from build123d import *

# Parameters (mm, degrees)
SKETCH_1_W                  = 320
SKETCH_1_H                  = 210
SKETCH_1_W_2                = 50
EXTRUDE_1_DEPTH             = 5
HOLE_WIZARD_M61_AT_2_COUNT  = 2
HOLE_WIZARD_M61_AT_2_PITCH  = 258
HOLE_WIZARD_M61_AT_3_COUNT  = 2
HOLE_WIZARD_M61_AT_3_PITCH  = 75
HOLE_WIZARD_M61_AT_4_COUNT  = 2
HOLE_WIZARD_M61_AT_4_PITCH  = 268.680107191
HOLE_WIZARD_M61_AT_5_COUNT  = 2
HOLE_WIZARD_M61_AT_5_PITCH  = 150
HOLE_WIZARD_M61_AT_6_COUNT  = 2
HOLE_WIZARD_M61_AT_6_PITCH  = 298.435922771
HOLE_WIZARD_M61_AT_7_COUNT  = 2
HOLE_WIZARD_M61_AT_7_PITCH  = 225
HOLE_WIZARD_M61_AT_8_COUNT  = 2
HOLE_WIZARD_M61_AT_8_PITCH  = 342.328789324
HOLE_WIZARD_M61_AT_9_COUNT  = 2
HOLE_WIZARD_M61_AT_9_PITCH  = 300
HOLE_WIZARD_M61_AT_10_COUNT = 2
HOLE_WIZARD_M61_AT_10_PITCH = 395.681690251
HOLE_WIZARD_M61_AT_11_COUNT = 2
HOLE_WIZARD_M61_AT_11_PITCH = 375
HOLE_WIZARD_M61_AT_12_COUNT = 2
HOLE_WIZARD_M61_AT_12_PITCH = 455.180184103
HOLE_WIZARD_M61_AT_13_COUNT = 2
HOLE_WIZARD_M61_AT_13_PITCH = 450
HOLE_WIZARD_M61_AT_14_COUNT = 2
HOLE_WIZARD_M61_AT_14_PITCH = 518.713793917
HOLE_WIZARD_M61_AT_15_COUNT = 2
HOLE_WIZARD_M61_AT_15_PITCH = 525
HOLE_WIZARD_M61_AT_16_COUNT = 2
HOLE_WIZARD_M61_AT_16_PITCH = 584.96922996
HOLE_WIZARD_M61_AT_17_COUNT = 2
HOLE_WIZARD_M61_AT_17_PITCH = 600
HOLE_WIZARD_M61_AT_18_COUNT = 2
HOLE_WIZARD_M61_AT_18_PITCH = 653.118672218
HOLE_WIZARD_M61_AT_19_COUNT = 2
HOLE_WIZARD_M61_AT_19_PITCH = 675
HOLE_WIZARD_M61_AT_20_COUNT = 2
HOLE_WIZARD_M61_AT_20_PITCH = 722.626459521
HOLE_WIZARD_M62_AT_2_COUNT  = 2
HOLE_WIZARD_M62_AT_2_PITCH  = 598
HOLE_WIZARD_M62_AT_3_COUNT  = 2
HOLE_WIZARD_M62_AT_3_PITCH  = 750
HOLE_WIZARD_M62_AT_4_COUNT  = 2
HOLE_WIZARD_M62_AT_4_PITCH  = 75
HOLE_WIZARD_M62_AT_5_COUNT  = 2
HOLE_WIZARD_M62_AT_5_PITCH  = 602.684826423
HOLE_WIZARD_M62_AT_6_COUNT  = 2
HOLE_WIZARD_M62_AT_6_PITCH  = 753.740671584
HOLE_WIZARD_M62_AT_7_COUNT  = 2
HOLE_WIZARD_M62_AT_7_PITCH  = 150
HOLE_WIZARD_M62_AT_8_COUNT  = 2
HOLE_WIZARD_M62_AT_8_PITCH  = 616.525749665
HOLE_WIZARD_M62_AT_9_COUNT  = 2
HOLE_WIZARD_M62_AT_9_PITCH  = 764.852927039


with BuildPart() as part:
    # Эскиз1 → Бобышка-Вытянуть1 (new body)
    with BuildSketch(Plane.XY):
        Polygon((0, 0), (750, 0), (750, 298), (0, 298), (-40, 298), (-40, 0), align=None)
        with Locations((394, 149)):
            Rectangle(SKETCH_1_W, SKETCH_1_H, mode=Mode.SUBTRACT)
        with Locations((189, 149)):
            Rectangle(SKETCH_1_W_2, SKETCH_1_H, mode=Mode.SUBTRACT)
    extrude(amount=EXTRUDE_1_DEPTH)

    # Эскиз2 → Зенковка для винта с потайной головкой и внутренним шестигранником M61 (revolve, cut)
    with BuildSketch(Plane(origin=(37.5, 278, 5), x_dir=(0, -1, 0), z_dir=(1, 0, 0))):
        Polygon((0, 0), (0, 5), (3.3, 5), (3.3, 3.555), (6.855, 0), align=None)
    hole_wizard_m61 = revolve(axis=Axis((37.5, 278, 11.35), (0, 0, -1)), mode=Mode.SUBTRACT)

    # Зенковка для винта с потайной головкой и внутренним шестигранником M61 at 2: Зенковка для винта с потайной головкой и внутренним шестигранником M61 ×2
    with Locations(*[(0, -i * HOLE_WIZARD_M61_AT_2_PITCH, 0) for i in range(1, HOLE_WIZARD_M61_AT_2_COUNT)]):
        add(hole_wizard_m61, mode=Mode.SUBTRACT)

    # Зенковка для винта с потайной головкой и внутренним шестигранником M61 at 3: Зенковка для винта с потайной головкой и внутренним шестигранником M61 ×2
    with Locations(*[(i * HOLE_WIZARD_M61_AT_3_PITCH, 0, 0) for i in range(1, HOLE_WIZARD_M61_AT_3_COUNT)]):
        add(hole_wizard_m61, mode=Mode.SUBTRACT)

    # Зенковка для винта с потайной головкой и внутренним шестигранником M61 at 4: Зенковка для винта с потайной головкой и внутренним шестигранником M61 ×2
    with Locations(*[Vector(0.2791423629542125, -0.9602497285624917, 0) * (i * HOLE_WIZARD_M61_AT_4_PITCH) for i in range(1, HOLE_WIZARD_M61_AT_4_COUNT)]):
        add(hole_wizard_m61, mode=Mode.SUBTRACT)

    # Зенковка для винта с потайной головкой и внутренним шестигранником M61 at 5: Зенковка для винта с потайной головкой и внутренним шестигранником M61 ×2
    with Locations(*[(i * HOLE_WIZARD_M61_AT_5_PITCH, 0, 0) for i in range(1, HOLE_WIZARD_M61_AT_5_COUNT)]):
        add(hole_wizard_m61, mode=Mode.SUBTRACT)

    # Зенковка для винта с потайной головкой и внутренним шестигранником M61 at 6: Зенковка для винта с потайной головкой и внутренним шестигранником M61 ×2
    with Locations(*[Vector(0.5026204573745305, -0.8645071866841928, 0) * (i * HOLE_WIZARD_M61_AT_6_PITCH) for i in range(1, HOLE_WIZARD_M61_AT_6_COUNT)]):
        add(hole_wizard_m61, mode=Mode.SUBTRACT)

    # Зенковка для винта с потайной головкой и внутренним шестигранником M61 at 7: Зенковка для винта с потайной головкой и внутренним шестигранником M61 ×2
    with Locations(*[(i * HOLE_WIZARD_M61_AT_7_PITCH, 0, 0) for i in range(1, HOLE_WIZARD_M61_AT_7_COUNT)]):
        add(hole_wizard_m61, mode=Mode.SUBTRACT)

    # Зенковка для винта с потайной головкой и внутренним шестигранником M61 at 8: Зенковка для винта с потайной головкой и внутренним шестигранником M61 ×2
    with Locations(*[Vector(0.6572628625373397, -0.7536614157094831, 0) * (i * HOLE_WIZARD_M61_AT_8_PITCH) for i in range(1, HOLE_WIZARD_M61_AT_8_COUNT)]):
        add(hole_wizard_m61, mode=Mode.SUBTRACT)

    # Зенковка для винта с потайной головкой и внутренним шестигранником M61 at 9: Зенковка для винта с потайной головкой и внутренним шестигранником M61 ×2
    with Locations(*[(i * HOLE_WIZARD_M61_AT_9_PITCH, 0, 0) for i in range(1, HOLE_WIZARD_M61_AT_9_COUNT)]):
        add(hole_wizard_m61, mode=Mode.SUBTRACT)

    # Зенковка для винта с потайной головкой и внутренним шестигранником M61 at 10: Зенковка для винта с потайной головкой и внутренним шестигранником M61 ×2
    with Locations(*[Vector(0.7581851963116828, -0.6520392688280476, 0) * (i * HOLE_WIZARD_M61_AT_10_PITCH) for i in range(1, HOLE_WIZARD_M61_AT_10_COUNT)]):
        add(hole_wizard_m61, mode=Mode.SUBTRACT)

    # Зенковка для винта с потайной головкой и внутренним шестигранником M61 at 11: Зенковка для винта с потайной головкой и внутренним шестигранником M61 ×2
    with Locations(*[(i * HOLE_WIZARD_M61_AT_11_PITCH, 0, 0) for i in range(1, HOLE_WIZARD_M61_AT_11_COUNT)]):
        add(hole_wizard_m61, mode=Mode.SUBTRACT)

    # Зенковка для винта с потайной головкой и внутренним шестигранником M61 at 12: Зенковка для винта с потайной головкой и внутренним шестигранником M61 ×2
    with Locations(*[Vector(0.823849572316137, -0.5668085057535025, 0) * (i * HOLE_WIZARD_M61_AT_12_PITCH) for i in range(1, HOLE_WIZARD_M61_AT_12_COUNT)]):
        add(hole_wizard_m61, mode=Mode.SUBTRACT)

    # Зенковка для винта с потайной головкой и внутренним шестигранником M61 at 13: Зенковка для винта с потайной головкой и внутренним шестигранником M61 ×2
    with Locations(*[(i * HOLE_WIZARD_M61_AT_13_PITCH, 0, 0) for i in range(1, HOLE_WIZARD_M61_AT_13_COUNT)]):
        add(hole_wizard_m61, mode=Mode.SUBTRACT)

    # Зенковка для винта с потайной головкой и внутренним шестигранником M61 at 14: Зенковка для винта с потайной головкой и внутренним шестигранником M61 ×2
    with Locations(*[Vector(0.8675304286814686, -0.4973841124440422, 0) * (i * HOLE_WIZARD_M61_AT_14_PITCH) for i in range(1, HOLE_WIZARD_M61_AT_14_COUNT)]):
        add(hole_wizard_m61, mode=Mode.SUBTRACT)

    # Зенковка для винта с потайной головкой и внутренним шестигранником M61 at 15: Зенковка для винта с потайной головкой и внутренним шестигранником M61 ×2
    with Locations(*[(i * HOLE_WIZARD_M61_AT_15_PITCH, 0, 0) for i in range(1, HOLE_WIZARD_M61_AT_15_COUNT)]):
        add(hole_wizard_m61, mode=Mode.SUBTRACT)

    # Зенковка для винта с потайной головкой и внутренним шестигранником M61 at 16: Зенковка для винта с потайной головкой и внутренним шестигранником M61 ×2
    with Locations(*[Vector(0.8974831035743466, -0.44104883947082196, 0) * (i * HOLE_WIZARD_M61_AT_16_PITCH) for i in range(1, HOLE_WIZARD_M61_AT_16_COUNT)]):
        add(hole_wizard_m61, mode=Mode.SUBTRACT)

    # Зенковка для винта с потайной головкой и внутренним шестигранником M61 at 17: Зенковка для винта с потайной головкой и внутренним шестигранником M61 ×2
    with Locations(*[(i * HOLE_WIZARD_M61_AT_17_PITCH, 0, 0) for i in range(1, HOLE_WIZARD_M61_AT_17_COUNT)]):
        add(hole_wizard_m61, mode=Mode.SUBTRACT)

    # Зенковка для винта с потайной головкой и внутренним шестигранником M61 at 18: Зенковка для винта с потайной головкой и внутренним шестигранником M61 ×2
    with Locations(*[Vector(0.9186691875800357, -0.3950277506594155, 0) * (i * HOLE_WIZARD_M61_AT_18_PITCH) for i in range(1, HOLE_WIZARD_M61_AT_18_COUNT)]):
        add(hole_wizard_m61, mode=Mode.SUBTRACT)

    # Зенковка для винта с потайной головкой и внутренним шестигранником M61 at 19: Зенковка для винта с потайной головкой и внутренним шестигранником M61 ×2
    with Locations(*[(i * HOLE_WIZARD_M61_AT_19_PITCH, 0, 0) for i in range(1, HOLE_WIZARD_M61_AT_19_COUNT)]):
        add(hole_wizard_m61, mode=Mode.SUBTRACT)

    # Зенковка для винта с потайной головкой и внутренним шестигранником M61 at 20: Зенковка для винта с потайной головкой и внутренним шестигранником M61 ×2
    with Locations(*[Vector(0.9340925606949639, -0.35703093431007527, 0) * (i * HOLE_WIZARD_M61_AT_20_PITCH) for i in range(1, HOLE_WIZARD_M61_AT_20_COUNT)]):
        add(hole_wizard_m61, mode=Mode.SUBTRACT)

    # Эскиз4 → Зенковка для винта с потайной головкой и внутренним шестигранником M62 (revolve, cut)
    with BuildSketch(Plane(origin=(-20, 224, 5), x_dir=(0, -1, 0), z_dir=(1, 0, 0))):
        Polygon((0, 0), (0, 5), (3.3, 5), (3.3, 3.555), (6.855, 0), align=None)
    hole_wizard_m62 = revolve(axis=Axis((-20, 224, 11.35), (0, 0, -1)), mode=Mode.SUBTRACT)

    # Зенковка для винта с потайной головкой и внутренним шестигранником M62 at 2: Зенковка для винта с потайной головкой и внутренним шестигранником M62 ×2
    with Locations(*[(i * HOLE_WIZARD_M62_AT_2_PITCH, 0, 0) for i in range(1, HOLE_WIZARD_M62_AT_2_COUNT)]):
        add(hole_wizard_m62, mode=Mode.SUBTRACT)

    # Зенковка для винта с потайной головкой и внутренним шестигранником M62 at 3: Зенковка для винта с потайной головкой и внутренним шестигранником M62 ×2
    with Locations(*[(i * HOLE_WIZARD_M62_AT_3_PITCH, 0, 0) for i in range(1, HOLE_WIZARD_M62_AT_3_COUNT)]):
        add(hole_wizard_m62, mode=Mode.SUBTRACT)

    # Зенковка для винта с потайной головкой и внутренним шестигранником M62 at 4: Зенковка для винта с потайной головкой и внутренним шестигранником M62 ×2
    with Locations(*[(0, -i * HOLE_WIZARD_M62_AT_4_PITCH, 0) for i in range(1, HOLE_WIZARD_M62_AT_4_COUNT)]):
        add(hole_wizard_m62, mode=Mode.SUBTRACT)

    # Зенковка для винта с потайной головкой и внутренним шестигранником M62 at 5: Зенковка для винта с потайной головкой и внутренним шестигранником M62 ×2
    with Locations(*[Vector(0.9922267390563397, -0.12444315289168138, 0) * (i * HOLE_WIZARD_M62_AT_5_PITCH) for i in range(1, HOLE_WIZARD_M62_AT_5_COUNT)]):
        add(hole_wizard_m62, mode=Mode.SUBTRACT)

    # Зенковка для винта с потайной головкой и внутренним шестигранником M62 at 6: Зенковка для винта с потайной головкой и внутренним шестигранником M62 ×2
    with Locations(*[Vector(0.9950371902099892, -0.09950371902099892, 0) * (i * HOLE_WIZARD_M62_AT_6_PITCH) for i in range(1, HOLE_WIZARD_M62_AT_6_COUNT)]):
        add(hole_wizard_m62, mode=Mode.SUBTRACT)

    # Зенковка для винта с потайной головкой и внутренним шестигранником M62 at 7: Зенковка для винта с потайной головкой и внутренним шестигранником M62 ×2
    with Locations(*[(0, -i * HOLE_WIZARD_M62_AT_7_PITCH, 0) for i in range(1, HOLE_WIZARD_M62_AT_7_COUNT)]):
        add(hole_wizard_m62, mode=Mode.SUBTRACT)

    # Зенковка для винта с потайной головкой и внутренним шестигранником M62 at 8: Зенковка для винта с потайной головкой и внутренним шестигранником M62 ×2
    with Locations(*[Vector(0.9699513772537904, -0.24329884044827513, 0) * (i * HOLE_WIZARD_M62_AT_8_PITCH) for i in range(1, HOLE_WIZARD_M62_AT_8_COUNT)]):
        add(hole_wizard_m62, mode=Mode.SUBTRACT)

    # Зенковка для винта с потайной головкой и внутренним шестигранником M62 at 9: Зенковка для винта с потайной головкой и внутренним шестигранником M62 ×2
    with Locations(*[Vector(0.9805806756909202, -0.19611613513818404, 0) * (i * HOLE_WIZARD_M62_AT_9_PITCH) for i in range(1, HOLE_WIZARD_M62_AT_9_COUNT)]):
        add(hole_wizard_m62, mode=Mode.SUBTRACT)


solid = part.part
The listing builds one solid part. Answer for the finished solid, in the listing's coordinates (mm). Round coordinates to 2 decimals unless told otherwise and drop trailing zeros. Order: outer loops, then holes, each group sorted by start corner. A loop starts at its lowest first (then second) coordinate and runs counter-clockwise, first axis right, second up. Notation, with made-up numbers: (-34, 59.25) -> (1, 59.25) arc R29 ccw to (1, 91.25) -> close; hole circle Ø4 at (-22, -30). An arc over 180 degrees is marked (long way). One line per item, written item: value.
Item 1: Given P1, Ø5.5, axis at x = -20, y = 224, coming from the +Z side; P2, Ø8.5, axis at x = -20, y = 74, coming from the +Z side (3 decimals); P3, Ø10.5, axis at x = 412.5, y = 278, coming from the +Z side (3 decimals); P4, Ø7.5, axis at x = 730, y = 74, coming from the +Z side (3 decimals), each flat-ended and moving along its own axis, determine where each tip first touches the part or whether it passes through.
Taken from the geometry:
P1: passes through
P2: stops at z = 2.395
P3: stops at z = 3.395
P4: stops at z = 1.895
Item 2: Find section C-C, the plane z = 2.9. State how many separate pieces and enclosed holes the cut face has, then the cut area to 3 significant figures.
Taken from the geometry:
separate pieces: 1
enclosed holes: 31
area: 156,000 mm2
Item 3: Find section B-B, the plane x = 514.5. Give the vertices of the cut face in (y, z).
Taken from the geometry:
outline: (0, 0) -> (44, 0) -> (44, 5) -> (0, 5) -> close; (254, 0) -> (298, 0) -> (298, 5) -> (254, 5) -> close
Item 4: Straight lines are drawn through the part: L1, parallel to X at y = 114, z = 2.7; L2, parallel to X at y = 149, z = 1.05; L3, parallel to Y at x = 406.5, z = 2.4. For each, find the intervals that lie inside material, in ascending order.
Taken from the geometry:
L1: x = -40 to 164, 214 to 234, 554 to 750
L2: x = -40 to -23.3, -16.7 to 164, 214 to 234, 554 to 574.7, 581.3 to 726.7, 733.3 to 750
L3: y = 0 to 44, 254 to 298
Item 5: For a pull along Y with two mould halves and no side action, classify faces 1 (the flat face through (349, 284, 0)), 2 (the conical face through (640.625, 18.375, 1.667)) as released by +Y, released by -Y, zero draft, split by the parting line, or undercut.
Taken from the geometry:
face 1: zero draft
face 2: undercut
Item 6: Find section A-A, the plane y = 124. Give the vertices of the cut face in (x, z), then the cut area to 3 significant figures.
Taken from the geometry:
outline: (-40, 0) -> (164, 0) -> (164, 5) -> (-40, 5) -> close; (214, 0) -> (234, 0) -> (234, 5) -> (214, 5) -> close; (554, 0) -> (750, 0) -> (750, 5) -> (554, 5) -> close
area: 2,100 mm2
